Could you check a few things on this model? Use its own coordinates, in mm. A direction names the side the tool comes from. Give positions to 0.01 mm unless a question says otherwise; leave off trailing zeros. Loops run counter-clockwise (first coordinate to the right, second up) from the corner with the lowest first, then second, coordinate; pieces in that order, holes last. Notation, with made-up numbers: M 36.25,27 L 64.25,27 A26 cw 64.25,43 Z; hole C 32.25,-35.75 d3. An arc over 180 degrees is marked long. Answer in a Markdown table with one row per item. Add a question column.
1. Thinking about a two-plate mould opening in X: for faces 3 (the cylindrical face through (-9.62, 181.94, -6.93)), 4 (the flat face through (-10, 99, 0)), 5 (the flat face through (9.25, 99, 0)), which applies, released by +X, released by -X, zero draft, split by the parting line, or undercut?
2. I'm going to push a flat-ended pin straight in: pin 1 Ø6 at (x, z) = (-3, 4.5) entering from -Y. Where does the tip first touch, or does it pass through?
3. Which directions (+Z, -Z, +X, -X, +Y, -Y) give clear straight access to the entire face, cutting with the end or side of a thin tool? Please do faces 1 (the flat face through (0, 104, -10)), 2 (the flat face through (0, 99, 9.25)).
4. If we section it at A-A on y = 30: List the corners of the cut face in (x, z) for me, then the cut area to 4 significant figures.
5. If we section it at C-C on z = -3.25: List the corners of the cut face in (x, y) for me, then the cut area to 3 significant figures.
6. I need wall thicknesses on line 1 along X through (y, z) = (179, 5.5); line 2 along Y through (x, z) = (9.7, 0). Which ranges of each line are inside material? Lowest first, please. Write a range as from..to.
7. If we section it at B-B on x = -2.5: List the corners of the cut face in (y, z) for me.
8. If we section it at D-D on y = 182.5: List the corners of the cut face in (x, z) for me.
Autodesk Inventor part; units mm, degrees
ref_plane "YZ Plane" through (0, 0, 0) normal (1, 0, 0) x (0, 1, 0)
ref_plane "XZ Plane" through (0, 0, 0) normal (0, 1, 0) x (-1, 0, 0)
ref_plane "XY Plane" through (0, 0, 0) normal (0, 0, 1) x (1, 0, 0)
sketch "Эскиз1" plane through (0, 0, 0) normal (0, 1, 0) x (-1, 0, 0)
  line L0 (-10, -10) -> (10, -10)
  line L1 (10, -10) -> (10, 10)
  line L2 (10, 10) -> (-10, 10)
  line L3 (-10, 10) -> (-10, -10)
  line L4 (-10, -10) -> (10, 10) construction
  line L5 (10, -10) -> (-10, 10) construction
  line L6 (-9.25, -9.25) -> (9.25, -9.25)
  line L7 (9.25, -9.25) -> (9.25, 9.25)
  line L8 (9.25, 9.25) -> (-9.25, 9.25)
  line L9 (-9.25, 9.25) -> (-9.25, -9.25)
  line L10 (-9.25, -9.25) -> (9.25, 9.25) construction
  line L11 (9.25, -9.25) -> (-9.25, 9.25) construction
  point P0 (0, 0)
  dimension "d0" = 20
  dimension "d1" = 20
  dimension "d2" = 18.5
  dimension "d3" = 18.5
extrude "Выдавливание1" add sketch "Эскиз1" along normal blind 200
sketch "Эскиз2" plane through (10, 0, 10) normal (1, 0, 0) x (0, 0, -1)
  line L0 (0, 0) -> (20, 0)
  line L1 (0, 0) -> (20, 11.547)
  line L2 (20, 0) -> (20, 200)
  line L3 (0, 0) -> (23.094, 0) construction
  line L4 (0, 0) -> (20, 0)
  line L5 (19.25, 0) -> (0.75, 0)
  line L6 (20, 11.547) -> (20, 0)
  point P0 (10, 0)
  dimension "d6" = 30
extrude "Выдавливание2" cut sketch "Эскиз2" against normal blind 200
sketch "Эскиз4" plane through (10, 200, 10) normal (1, 0, 0) x (0, 0, -1)
  circle A0 centre (10, -15.1881) radius 7.5
  point P0 (10, -200)
  dimension "d9" = 15
extrude "Выдавливание3" cut sketch "Эскиз4" against normal blind 124
properties part number "опора кинематик стенд"
Results:
| question | item | result |
|---|---|---|
| 1 | face 3 | zero draft |
| 1 | face 4 | released by -X |
| 1 | face 5 | undercut |
| 2 | pin 1 | through |
| 3 | face 1 | -Z, +X, -X, +Y, -Y |
| 3 | face 2 | +Y, -Y |
| 4 | outline | M -10,-10 L 10,-10 L 10,10 L -10,10 Z; hole M -9.25,-9.25 L 9.25,-9.25 L 9.25,9.25 L -9.25,9.25 Z |
| 4 | area | 57.75 mm2 |
| 5 | outline | M -10,7.65 L -9.25,7.65 L -9.25,178.05 L -10,178.05 Z; M -10,191.57 L -9.25,191.57 L -9.25,200 L -10,200 Z; M 9.25,7.65 L 10,7.65 L 10,178.05 L 9.25,178.05 Z; M 9.25,191.57 L 10,191.57 L 10,200 L 9.25,200 Z |
| 5 | area | 268 mm2 |
| 6 | line 1 | -10..-9.25, 9.25..10 |
| 6 | line 2 | 5.77..177.31, 192.31..200 |
| 7 | outline | M 0,10 L 0.43,9.25 L 200,9.25 L 200,10 Z; M 11.11,-9.25 L 11.55,-10 L 200,-10 L 200,-9.25 Z |
| 8 | outline | M -10,-10 L 10,-10 L 10,-7.13 L 9.25,-7.13 L 9.25,-9.25 L -9.25,-9.25 L -9.25,-7.13 L -10,-7.13 Z; M -10,7.13 L -9.25,7.13 L -9.25,9.25 L 9.25,9.25 L 9.25,7.13 L 10,7.13 L 10,10 L -10,10 Z |
